For this review, use the dimensioned drawing (mm, ordinates from the lowest corner) and the shaded views. Coordinates: 2 decimals unless noted, no trailing zeros. Loops run counter-clockwise (first coordinate to the right, second up) from the corner with the lowest first, then second, coordinate; pieces in that order, holes last. Notation, with made-up numbers: M 38,22.5 L 43,22.5 A15 cw 43,39.5 Z; hole C -38.5,-29.75 d5. An arc over 180 degrees is marked long. Write item = value, one per line.
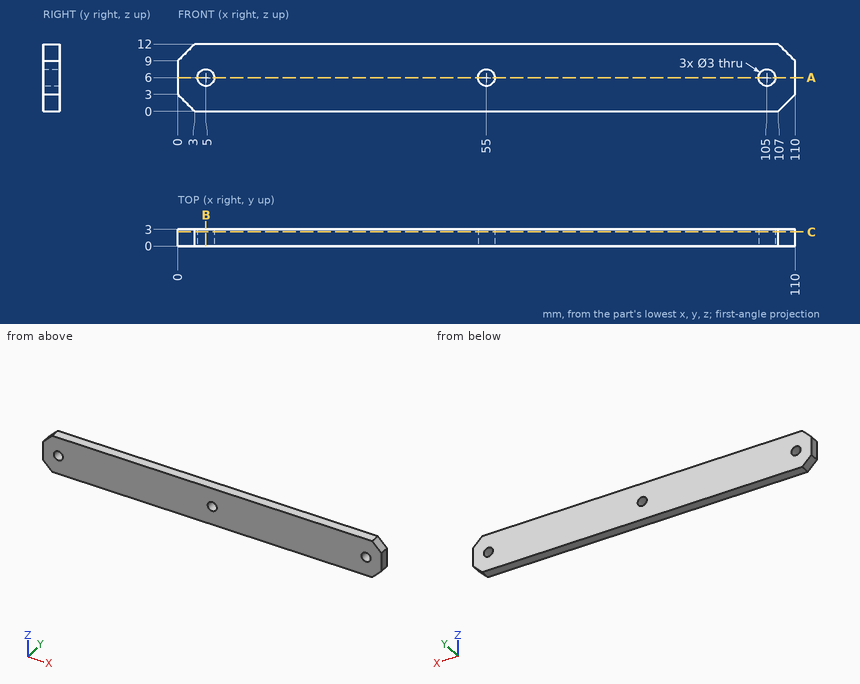
Q1. Add section C-C (y = 2.55). Write out the cut boundary in (x, z), and give its area (3 significant figures).
Solved:
outline = M 0,3 L 3,0 L 107,0 L 110,3 L 110,9 L 107,12 L 3,12 L 0,9 Z; hole C 5,6 d3; hole C 55,6 d3; hole C 105,6 d3
area = 1,280 mm²
Q2. Add section A-A (z = 6). Write out the cut boundary in (x, y), and give its area (3 significant figures).
Solved:
outline = M 0,0 L 3.5,0 L 3.5,3 L 0,3 Z; M 6.5,0 L 53.5,0 L 53.5,3 L 6.5,3 Z; M 56.5,0 L 103.5,0 L 103.5,3 L 56.5,3 Z; M 106.5,0 L 110,0 L 110,3 L 106.5,3 Z
area = 303 mm²
Q3. For line 1 along X through (y, z) = (2.3, 6); line 2 along X through (y, z) = (2, 7); line 3 along Z through (x, y) = (105, 0.85), list the stretches that pass through material, from the lowest coordinate up.
Solved:
line_1 = 0 to 3.5, 6.5 to 53.5, 56.5 to 103.5, 106.5 to 110
line_2 = 0 to 3.88, 6.12 to 53.88, 56.12 to 103.88, 106.12 to 110
line_3 = 0 to 4.5, 7.5 to 12
Q4. Add section B-B (x = 5). Write out the cut boundary in (y, z).
Solved:
outline = M 0,0 L 3,0 L 3,4.5 L 0,4.5 Z; M 0,7.5 L 3,7.5 L 3,12 L 0,12 Z
